Autodesk Inventor part; units mm, degrees
ref_plane "YZ Plane" through (0, 0, 0) normal (1, 0, 0) x (0, 1, 0)
ref_plane "XZ Plane" through (0, 0, 0) normal (0, 1, 0) x (-1, 0, 0)
ref_plane "XY Plane" through (0, 0, 0) normal (0, 0, 1) x (1, 0, 0)
sketch "Sketch1" plane through (0, 0, 0) normal (0, 0, 1) x (1, 0, 0)
  ellipse E0 centre (0, 0) end of major axis (95, 0) minor radius 80 (0, -80) -> (0, 80) ccw
  ellipse E1 centre (0, 0) end of major axis (75, 0) minor radius 60 (0, -60) -> (0, 60) ccw
  line L0 (0, 80) -> (0, 73)
  line L1 (0, 73) -> (-6, 73)
  line L2 (-6, 73) -> (-6, 67)
  line L3 (-6, 67) -> (0, 67)
  line L4 (0, 67) -> (0, 60)
  line L5 (75, 0) -> (95, 0) construction
  line L6 (0, -73) -> (-6, -73)
  line L7 (-6, -73) -> (-6, -67)
  line L8 (-6, -67) -> (0, -67)
  line L9 (0, -60) -> (0, -67)
  line L10 (0, -73) -> (0, -80)
  line L11 (85, -35.7275) -> (85, 35.7275) construction
  line L12 (85, -3) -> (85, 3)
  line L13 (85, 3) -> (94.9332, 3)
  line L14 (85, -3) -> (94.9332, -3)
  point P0 (85, 0)
  dimension "d0" = 80
  dimension "d2" = 75
  dimension "d3" = 60
  dimension "d4" = 95
  dimension "d6" = 6
  dimension "d7" = 6
extrude "Extrusion1" add sketch "Sketch1" along normal blind 6 contours L10 L6 L7 L8 L9 E1 L4 L3 L2 L1 L0 E0 L13 L12 L14
properties part number "Arch Rear Inner" material "Plywood, Sheathing"
The model under review builds one solid part; all positions refer to its coordinate system, in mm. A direction names the side the tool comes from. Coordinates: 2 decimals unless noted, no trailing zeros. Use a Markdown table: item, result. Add a question column.
1. Clearance check with flat-ended pins moving along their axes: pin 1 Ø3 at (x, z) = (-3, 4) entering from -Y; pin 2 Ø1.8 at (x, z) = (87.5, 3) entering from -Y; pin 3 Ø1.8 at (y, z) = (0, 3) entering from +X; pin 4 Ø8 at (x, y) = (77.5, -41) entering from -Z. State where each tip first meets the part, or that it passes through.
2. Draft analysis for pull direction Y (two halves, no side actions). For faces 1 (the face through (0, -63, 3)), 2 (the face through (-3, -73, 3)), 3 (the face through (85, 0, 3)), 4 (the face through (-6, 70, 3)), state which applies: pulls with the +Y half, pulls with the -Y half, needs draft (parallel to the pull), parting line crosses it, or undercut.
3. Machinability: for faces 5 (the face through (-3, 73, 3)), 6 (the face through (0, 64, 3)), 7 (the face through (90, 3, 3)), which of the approach directions +Z, -Z, +X, -X, +Y, -Y give a long, thin tool a straight path to every point of the face, cutting with its end or side? Answer none if there is none.
4. To check wall thickness, follow line 1 (Y direction, x = 1, z = 2.85); line 2 (Y direction, x = 89, z = 3.15); line 3 (X direction, y = 21, z = 4.9). State the ranges of each line that lie inside material, in increasing order.
Returned:
| question | item | result |
|---|---|---|
| 1 | pin 1 | stops at y = -73 |
| 1 | pin 2 | stops at y = -32.89 |
| 1 | pin 3 | stops at x = 85 |
| 1 | pin 4 | stops at z = 0 |
| 2 | face 1 | undercut |
| 2 | face 2 | pulls with the -Y half |
| 2 | face 3 | undercut |
| 2 | face 4 | needs draft |
| 3 | face 5 | +Z, -Z, -X, +Y |
| 3 | face 6 | +Z, -Z, -X |
| 3 | face 7 | +Z, -Z, +X |
| 4 | line 1 | y = -80 to -59.99, 59.99 to 80 |
| 4 | line 2 | y = -27.98 to -3, 3 to 27.98 |
| 4 | line 3 | x = 70.26 to 91.67 |
